Study the drawing (mm; zero at the part's minimum x, y, z) and answer. Coordinates: 2 decimals unless noted, no trailing zeros. Loops run counter-clockwise (first coordinate to the right, second up) from the corner with the lowest first, then second, coordinate; pieces in that order, holes last.
Q1. Section D-D (y = 25) is taken. Give the vertices of the cut face in (x, z), then the cut area to 3 significant figures.
Q2. Section A-A (z = 6) is taken. Give the vertices of the cut face in (x, y).
Q3. Flat-ended cylindrical pins translate along their axes: P1, Ø3, axis at y = 25, z = 6, coming from the +X side; P2, Ø4, axis at x = 6, z = 6, coming from the -Y side. Find the tip coordinate at first contact, or state that the pin passes through.
Q4. The mould has two halves that part along Z. Classify the marked faces 1, 2 and 3: pulls with the +Z half, pulls with the -Z half, needs draft (parallel to the pull), parting line crosses it, or undercut.
Q5. Section C-C (y = 5) is taken. Give the vertices of the cut face in (x, z).
Q6. Straight lines are drawn through the part: line 1 (Z direction, x = 6, y = 10.5); line 2 (X direction, y = 9.5, z = 6.5); line 3 (Z direction, x = 7, y = 2). For each, find the intervals that lie inside material, in ascending order.
Q7. Section B-B (x = 6) is taken. Give the vertices of the cut face in (y, z).
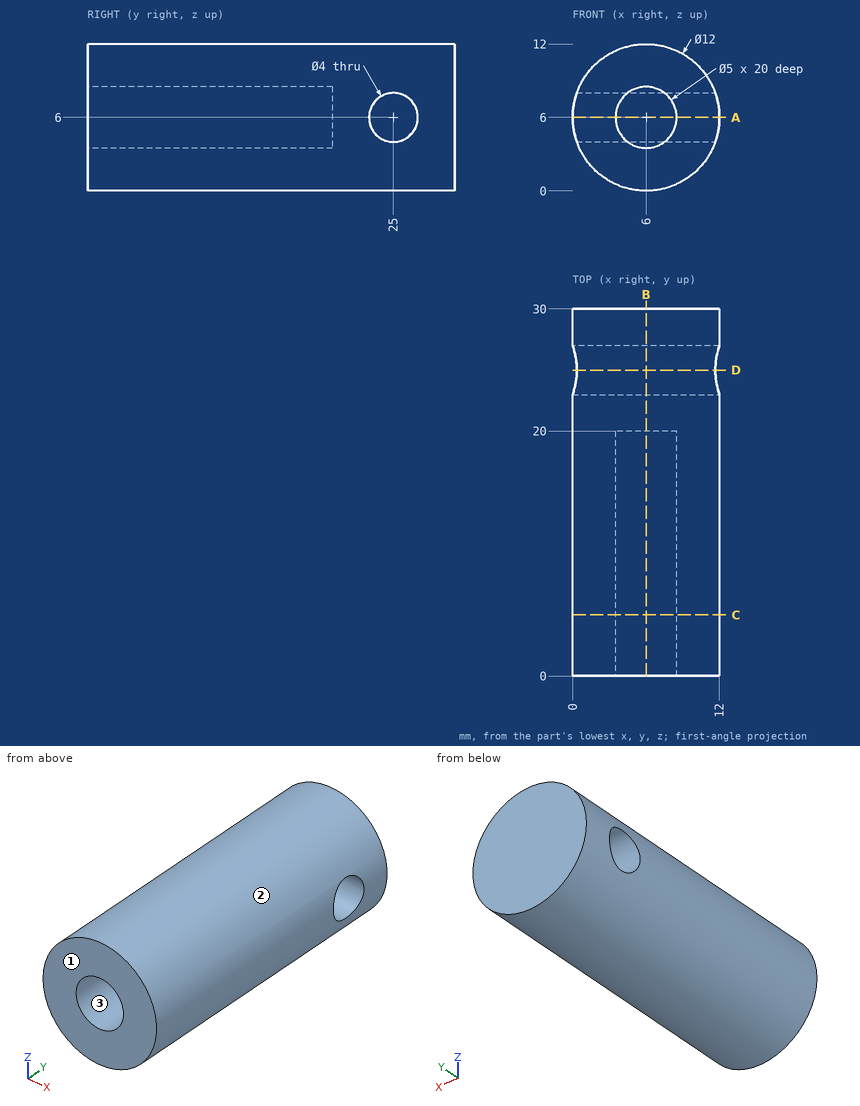
Numbers:
1. outline: (0.34, 4) arc R6 ccw to (11.66, 4) - close; (0.34, 8) - (11.66, 8) arc R6 ccw to start
1. area: 66.0 mm2
2. outline: (0, 0) - (3.5, 0) - (3.5, 20) - (8.5, 20) - (8.5, 0) - (12, 0) - (12, 23) - (0, 23) - close; (0, 27) - (12, 27) - (12, 30) - (0, 30) - close
3. P1: passes through
3. P2: stops at y = 20
4. face 1: needs draft
4. face 2: parting line crosses it
4. face 3: undercut
5. outline: circle Ø12 at (6, 6); hole circle Ø5 at (6, 6)
6. line 1: z = 0 to 3.5, 8.5 to 12
6. line 2: x = 0.02 to 3.55, 8.45 to 11.98
6. line 3: z = 0.08 to 3.71, 8.29 to 11.92
7. outline: (0, 0) - (30, 0) - (30, 12) - (0, 12) - (0, 8.5) - (20, 8.5) - (20, 3.5) - (0, 3.5) - close; hole circle Ø4 at (25, 6)
